Autodesk Inventor part; units mm, degrees
ref_plane "YZ Plane" through (0, 0, 0) normal (1, 0, 0) x (0, 1, 0)
ref_plane "XZ Plane" through (0, 0, 0) normal (0, 1, 0) x (-1, 0, 0)
ref_plane "XY Plane" through (0, 0, 0) normal (0, 0, 1) x (1, 0, 0)
sketch "スケッチ1" plane through (0, 0, 0) normal (0, 0, 1) x (1, 0, 0)
  circle A0 centre (0, 0) radius 10
  circle A1 centre (0, 0) radius 1.6
  circle A2 centre (0, 0) radius 7 construction
  circle A3 centre (0, 7) radius 0.8
  line L0 (0, 7) -> (0, 0) construction
  circle A4 centre (-4.9497, 4.9497) radius 0.8
  circle A5 centre (-7, 0) radius 0.8
  circle A6 centre (-4.9497, -4.9497) radius 0.8
  circle A7 centre (0, -7) radius 0.8
  circle A8 centre (4.9497, -4.9497) radius 0.8
  circle A9 centre (7, 0) radius 0.8
  circle A10 centre (4.9497, 4.9497) radius 0.8
  dimension "d2" = 14
  dimension "d0" = 20
  dimension "d1" = 3.2
  dimension "d3" = 1.6
  dimension "d6" = 360
extrude "押し出し1" add sketch "スケッチ1" along normal blind 2
sketch "スケッチ2" plane through (0, 0, 2) normal (0, 0, 1) x (1, 0, 0)
  circle A0 centre (0, 0) radius 1.6
  circle A1 centre (0, 0) radius 10
  circle A2 centre (0, 0) radius 5
  dimension "d10" = 10
extrude "押し出し2" add sketch "スケッチ2" along normal blind 1 contours A2
sketch "スケッチ3" plane through (0, 0, 0) normal (0, 0, -1) x (-1, 0, 0)
  circle A0 centre (0, 0) radius 1.6
  circle A1 centre (0, 0) radius 10
  circle A2 centre (0, 0) radius 5
  dimension "d13" = 10
extrude "押し出し3" add sketch "スケッチ3" along normal blind 1 contours A2
sketch "スケッチ4" plane through (0, 0, -1) normal (0, 0, -1) x (-1, 0, 0)
  circle A0 centre (0, 0) radius 1.6
  circle A1 centre (0, 0) radius 5
  circle A2 centre (0, 0) radius 3
  dimension "d16" = 6
extrude "押し出し4" cut sketch "スケッチ4" against normal blind 3 contours A2
properties part number "アルミローハイトサーボホーン" material "アルミニウム 2014-T4"
Could you check a few things on this model? Use its own coordinates, in mm. A direction names the side the tool comes from. Give positions to 0.01 mm unless a question says otherwise; leave off trailing zeros. Write each loop counter-clockwise with the first axis right and the second up, starting at its lowest first coordinate (ties: lowest second). Pieces come first, ordered by that corner, then holes. Notation, with made-up numbers: (31, 14) - (36, 14) arc R19 cw to (36, 32) - close; hole circle Ø6 at (24, -30.5). An arc over 180 degrees is marked (long way). Use CSV: the item, a comma, the result in double quotes. Start each with the question number.
Item 1: For faces 4 (the face through (-7.8, 0, 1)), 5 (the face through (-1.08, 4.88, 2.49)), 6 (the face through (-1.3, -1.3, 2)), which set-ups out of +Z, -Z, +X, -X, +Y, -Y let a thin tool reach every point of the face, with its end or its side?
Item 2: If we mould it in two halves opening along X, with no side actions, what happens to faces 1 (the face through (1.08, 4.88, -0.49)), 2 (the face through (3, 0, 0)), 3 (the face through (2, 5, 2))? For each: pulls with the +X half, pulls with the -X half, needs draft (parallel to the pull), parting line crosses it, or undercut.
Item 3: If I drill on line 1 along Y through (x, z) = (4.25, 1.1); line 2 along X through (y, z) = (4.5, 1.75), over which ranges is the centre line in solid material (lowest first)?
Item 4: I'm going to push flat-ended pins straight in: pin 1 (1.4 mm diameter, centred on x = 4.95, y = -4.95, fed in from +Z); pin 2 (1.8 mm diameter, centred on x = -4.95, y = 4.95, fed in from -Z); pin 3 (3 mm diameter, centred on x = 0.5, y = 0, fed in from -Z); pin 4 (2.5 mm diameter, centred on x = -4.95, y = -4.95, fed in from +Z). Where does each tip first touch, or does it pass through?
Item 5: I want a section at C-C, the plane y = 5.5. Please give me the cut outline in (x, z), then the cut area to 3 significant figures.
Item 6: I want a section at A-A, the plane x = 0. Please give me the cut outline in (y, z), then the cut area to 3 significant figures.
Item 7: I want a section at D-D, the plane z = 0.95. Give the number of separate pieces and of enclosed holes in the cut face, then the cut area to 3 significant figures.
Findings:
1,face 4,"+Z, -Z"
1,face 5,"+Z"
1,face 6,"-Z"
2,face 1,"parting line crosses it"
2,face 2,"undercut"
2,face 3,"needs draft"
3,line 1,"y = -9.05 to -5.34, -4.56 to 4.56, 5.34 to 9.05"
3,line 2,"x = -8.93 to -5.61, -4.29 to 4.29, 5.61 to 8.93"
4,pin 1,"passes through"
4,pin 2,"stops at z = 0"
4,pin 3,"stops at z = 2"
4,pin 4,"stops at z = 2"
5,outline,"(-8.35, 0) - (-5.53, 0) - (-5.53, 2) - (-8.35, 2) - close; (-4.37, 0) - (4.37, 0) - (4.37, 2) - (-4.37, 2) - close; (5.53, 0) - (8.35, 0) - (8.35, 2) - (5.53, 2) - close"
5,area,"28.8 mm2"
6,outline,"(-10, 0) - (-7.8, 0) - (-7.8, 2) - (-10, 2) - close; (-6.2, 0) - (-5, 0) - (-5, -1) - (-3, -1) - (-3, 2) - (-1.6, 2) - (-1.6, 3) - (-5, 3) - (-5, 2) - (-6.2, 2) - close; (1.6, 2) - (3, 2) - (3, -1) - (5, -1) - (5, 0) - (6.2, 0) - (6.2, 2) - (5, 2) - (5, 3) - (1.6, 3) - close; (7.8, 0) - (10, 0) - (10, 2) - (7.8, 2) - close"
6,area,"32.4 mm2"
7,separate pieces,"1"
7,enclosed holes,"9"
7,area,"270 mm2"
